Input: part model. Units: mm. Frame: model coordinates. A direction names the side the tool comes from. Coordinates: 2 decimals unless noted, no trailing zeros. Order: outer loops, then holes, each group sorted by start corner. A loop starts at its lowest first (then second) coordinate and runs counter-clockwise, first axis right, second up. Notation, with made-up numbers: (71.25, 9.25) -> (128.25, 9.25) arc R13 cw to (128.25, 25.25) -> close; hole circle Ø8 at (-13, -28). An arc over 180 degrees is marked (long way). Write each question's results on one line, items separated by ' | '.
Autodesk Inventor part; units mm, degrees
ref_plane "Plano de trabajo3" through (-215, 140, 0) normal (0, 1, 0) x (1, 0, 0)
ref_plane "YZ Plane" through (0, 0, 0) normal (1, 0, 0) x (0, 1, 0)
ref_plane "XZ Plane" through (0, 0, 0) normal (0, 1, 0) x (-1, 0, 0)
sketch "Boceto1" plane through (0, 0, 0) normal (0, 0, 1) x (1, 0, 0)
  line L0 (-215, 142.5) -> (215, 142.5)
  line L1 (215, 142.5) -> (215, -142.5)
  line L2 (215, -142.5) -> (-215, -142.5)
  line L3 (-215, -142.5) -> (-215, 142.5)
  line L4 (-215, 142.5) -> (215, -142.5) construction
  line L5 (215, 142.5) -> (-215, -142.5) construction
  point P0 (0, 0)
  dimension "d0" = 430
  dimension "d1" = 285
extrude "Extrusión1" add sketch "Boceto1" along normal blind 3
sketch "Boceto2" plane through (0, 0, 3) normal (0, 0, 1) x (1, 0, 0)
  line L0 (-50, -12.5) -> (50, -12.5)
  line L1 (50, -12.5) -> (50, 12.5)
  line L2 (50, 12.5) -> (-50, 12.5)
  line L3 (-50, 12.5) -> (-50, -12.5)
  line L4 (-50, -12.5) -> (50, 12.5) construction
  line L5 (50, -12.5) -> (-50, 12.5) construction
  point P0 (0, 0)
  dimension "d4" = 100
  dimension "d5" = 25
extrude "Extrusión2" add sketch "Boceto2" along normal blind 5
sketch "Boceto3" plane through (50, -12.5, 3) normal (1, 0, 0) x (0, 0, -1)
  line L0 (-5, 0) -> (-5, 12.5)
  arc A0 (-10, 17.5) -> (-10, 7.5) centre (-10, 12.5) ccw
  circle A1 centre (-10, 12.5) radius 2.5
  line L1 (-5, 0) -> (-5, 25)
  line L2 (-10, 7.5) -> (-5, 7.5)
  line L3 (-5, 7.5) -> (-5, 17.5)
  line L4 (-5, 17.5) -> (-10, 17.5)
  point P0 (3, 12.5)
  dimension "d10" = 5
extrude "Extrusión3" add sketch "Boceto3" against normal blind 100
sketch "Boceto13" plane through (0, 0, 3) normal (0, 0, 1) x (1, 0, 0)
  line L0 (215, 142.5) -> (-215, 142.5)
  line L1 (-215, 142.5) -> (-210, 142.5)
  line L2 (-210, 142.5) -> (-210, 137.5)
  line L3 (-210, 137.5) -> (-215, 137.5)
  line L4 (-215, 137.5) -> (-215, 142.5)
  line L5 (215, -142.5) -> (215, 142.5)
  line L6 (215, 142.5) -> (210, 142.5)
  line L7 (210, 142.5) -> (210, 137.5)
  line L8 (210, 137.5) -> (215, 137.5)
  line L9 (215, 137.5) -> (215, 142.5)
  line L10 (-215, -142.5) -> (215, -142.5)
  line L11 (215, -142.5) -> (210, -142.5)
  line L12 (210, -142.5) -> (210, -137.5)
  line L13 (210, -137.5) -> (215, -137.5)
  line L14 (215, -137.5) -> (215, -142.5)
  line L15 (-215, -142.5) -> (-210, -142.5)
  line L16 (-210, -142.5) -> (-210, -137.5)
  line L17 (-210, -137.5) -> (-215, -137.5)
  line L18 (-215, -137.5) -> (-215, -142.5)
  point P0 (0, 0)
  dimension "d39" = 5
  dimension "d40" = 5
  dimension "d41" = 5
  dimension "d42" = 5
  dimension "d43" = 5
  dimension "d44" = 5
  dimension "d45" = 5
  dimension "d46" = 5
extrude "Extrusión10" add sketch "Boceto13" along normal blind 10
sketch "Boceto16" plane through (-215, -142.5, 0) normal (-1, 0, 0) x (0, 0, 1)
  line L0 (13, 5) -> (13, 0)
  circle A0 centre (10.5, 2.5) radius 2.5
  line L1 (13, 285) -> (13, 280)
  circle A1 centre (10.5, 282.5) radius 2.5
  point P0 (0, 142.5)
extrude "Extrusión13" add sketch "Boceto16" along normal blind 45
sketch "Boceto17" plane through (215, -142.5, 0) normal (1, 0, 0) x (0, 0, -1)
  line L0 (-13, 280) -> (-13, 285)
  circle A0 centre (-10.5, 282.5) radius 2.5
  line L1 (-13, 0) -> (-13, 5)
  circle A1 centre (-10.5, 2.5) radius 2.5
  point P0 (0, 142.5)
extrude "Extrusión14" add sketch "Boceto17" along normal blind 45
ref_plane "Plano de trabajo3" through (-215, 140, 0) normal (0, 1, 0) x (1, 0, 0)
sketch "Boceto18" plane through (-215, 140, 0) normal (0, 1, 0) x (1, 0, 0)
  line L0 (475, -13) -> (475, -8)
  line L1 (475, -10.5) -> (470.5, -10.5)
  line L2 (470.5, -10.5) -> (470.5, -13)
  line L3 (430, -13) -> (475, -13)
  line L4 (470, -13.5) -> (471, -13.5)
  line L5 (471, -13.5) -> (471, -12.5)
  line L6 (471, -12.5) -> (470, -12.5)
  line L7 (470, -12.5) -> (470, -13.5)
  line L8 (470, -13.5) -> (471, -12.5) construction
  line L9 (471, -13.5) -> (470, -12.5) construction
  line L10 (-45, -8) -> (-45, -13)
  line L11 (-45, -10.5) -> (-38.08, -10.5)
  line L12 (-38.08, -10.5) -> (-38.08, -13)
  line L13 (0, -13) -> (-45, -13)
  line L14 (-38.58, -13.5) -> (-37.58, -13.5)
  line L15 (-37.58, -13.5) -> (-37.58, -12.5)
  line L16 (-37.58, -12.5) -> (-38.58, -12.5)
  line L17 (-38.58, -12.5) -> (-38.58, -13.5)
  line L18 (-38.58, -13.5) -> (-37.58, -12.5) construction
  line L19 (-37.58, -13.5) -> (-38.58, -12.5) construction
  point P0 (215, 0)
  point P1 (470, -13)
  point P2 (471, -13)
  dimension "d68" = 4.5
  dimension "d69" = 1
  dimension "d70" = 1
  dimension "d72" = 6.92
  dimension "d73" = 1
  dimension "d74" = 1
revolve "Revolución1" cut sketch "Boceto18" angle 360 about axis through (260, 140, 10.5) along (-1, 0, 0) contours L3 L2 L6 L5 | L3 L7 L6 L2 | L17 L16 L12 L13 | L13 L15 L14 L17 | L16 L15 L13 L12
ref_plane "Plano de trabajo4" through (210, -140, 3) normal (0, 1, 0) x (1, 0, 0)
sketch "Boceto19" plane through (210, -140, 3) normal (0, 1, 0) x (1, 0, 0)
  line L0 (50, -10) -> (50, -5)
  line L1 (50, -7.5) -> (45.5, -7.5)
  line L2 (45.5, -7.5) -> (45.5, -10)
  line L3 (5, -10) -> (50, -10)
  line L4 (46, -10.5) -> (45, -10.5)
  line L5 (45, -10.5) -> (45, -9.5)
  line L6 (45, -9.5) -> (46, -9.5)
  line L7 (46, -9.5) -> (46, -10.5)
  line L8 (46, -10.5) -> (45, -9.5) construction
  line L9 (45, -10.5) -> (46, -9.5) construction
  line L10 (-470, -5) -> (-470, -10)
  line L11 (-470, -7.5) -> (-463.08, -7.5)
  line L12 (-463.08, -7.5) -> (-463.08, -10)
  line L13 (-462.58, -10) -> (-462.58, -5)
  line L14 (-463.58, -10.5) -> (-462.58, -10.5)
  line L15 (-462.58, -10.5) -> (-462.58, -9.5)
  line L16 (-462.58, -9.5) -> (-463.58, -9.5)
  line L17 (-463.58, -9.5) -> (-463.58, -10.5)
  line L18 (-463.58, -10.5) -> (-462.58, -9.5) construction
  line L19 (-462.58, -10.5) -> (-463.58, -9.5) construction
  point P0 (-210, 3)
  dimension "d76" = 4.5
  dimension "d77" = 1
  dimension "d78" = 1
  dimension "d79" = 6.92
  dimension "d80" = 1
revolve "Revolución2" cut sketch "Boceto19" angle 360 about axis through (260, -140, 10.5) along (-1, 0, 0) contours L7 L4 L5 L3 | L3 L2 L6 L7 | L3 L5 L6 L2 | L15 L14 L17 L16 L13
sketch "Sketch20" plane through (0, 0, 0) normal (0, 0, -1) x (-1, 0, 0)
  line L0 (215, 142.5) -> (215, -142.5)
  line L1 (215, -142.5) -> (-215, -142.5)
  line L2 (-215, 142.5) -> (215, 142.5)
  line L3 (-215, -142.5) -> (-215, 142.5)
  point P0 (0, 0)
extrude "Extrusion15" add sketch "Sketch20" along normal blind 3
sketch "Sketch22" plane through (0, 0, -3) normal (0, 0, -1) x (-1, 0, 0)
  line L0 (0, 0) -> (0, 23) construction
  circle A0 centre (0, 23) radius 3
  dimension "d84" = 23
  dimension "d85" = 6
extrude "Extrusion16" cut sketch "Sketch22" against normal blind 6
properties part number "Bandeja"
(1) Reachability of faces 1 (the face through (1, 0, 18)), 2 (the face through (-50, 0, 7)), 3 (the face through (50, 0, 7)) from +Z, -Z, +X, -X, +Y, -Y: full face, straight path, thin tool, end or side. Return the list, or none.
Return value:
face 1: +Z, +X, -X | face 2: +Z, -X, +Y, -Y | face 3: +Z, +X, +Y, -Y
(2) Pin query (flat end, axial travel): P1, Ø4, axis at x = -7, z = 11.5, coming from the -Y side; P2, Ø12, axis at y = 13, z = 12.5, coming from the -X side; P3, Ø2.5, axis at y = 140, z = 6.5, coming from the -X side. Return the tip coordinate at first contact, or that it passes through.
Return value:
P1: y = -5 | P2: x = -50 | P3: x = -215
(3) Cut plane C-C, the plane x = 136. Return loops of the section in (y, z).
Return value:
outline: (-142.5, -3) -> (142.5, -3) -> (142.5, 3) -> (-142.5, 3) -> close
(4) Line query: line 1 along Y through (x, z) = (0, 1.3); line 2 along Y through (x, z) = (16, 13); line 3 along Z through (x, y) = (152, -78.5). Output: solid intervals per line, ascending. Write a range as from..to.
Return value:
line 1: -142.5..20, 26..142.5 | line 2: -5..-2.5, 2.5..5 | line 3: -3..3
(5) Cut plane A-A, the plane x = 8.5. Return loops of the section in (y, z), plus the area to 3 significant figures.
Return value:
outline: (-142.5, -3) -> (142.5, -3) -> (142.5, 3) -> (12.5, 3) -> (12.5, 8) -> (5, 8) -> (5, 13) arc R5 ccw to (-5, 13) -> (-5, 8) -> (-12.5, 8) -> (-12.5, 3) -> (-142.5, 3) -> close; hole circle Ø5 at (0, 13) | area: 1,900 mm2
(6) Cut plane B-B, the plane y = 109. Return loops of the section in (x, z).
Return value:
outline: (-215, -3) -> (215, -3) -> (215, 3) -> (-215, 3) -> close
